Geometry check sheet. Reference: the model listing, model coordinates, mm. Face numbers are marked on the shaded views. A direction names the side the tool comes from. Coordinates: 2 decimals unless noted, no trailing zeros. Write each loop counter-clockwise with the first axis right and the second up, starting at its lowest first coordinate (ties: lowest second). Pieces come first, ordered by that corner, then holes. Notation, with made-up numbers: (-14.5, -18) -> (39.5, -18) arc R18 cw to (39.5, -2) -> close; hole circle Ø6 at (-39, 3.25). An arc over 180 degrees is marked (long way). Use a Markdown table: item, result.
```python
from build123d import *

# Parameters (mm, degrees)
SKETCH1_R                       = 1.975
PCB_DEPTH                       = 0.825
SKETCH7_R                       = 1.475
INNER_HOLES_DEPTH               = 1
INNER_HOLES_DEPTH_BACK          = 2.65
SKETCH8_W                       = 10
SKETCH8_H                       = 4.35
CONNECTOR_DEPTH                 = 2.6
SKETCH9_W                       = 4.3
SKETCH9_H                       = 2
TOP_COMPONENT_DEPTH             = 2.255
SKETCH10_W                      = 5.75
SKETCH10_H                      = 5
SIDE_COMPONENTS_DEPTH           = 1.1
SKETCH11_W                      = 10.5
SKETCH11_H                      = 17
CENTRAL_COMPONENTS_DEPTH        = 1.825
SKETCH12_W                      = 5.575
SKETCH12_H                      = 5
TOP_AND_BOTTOM_COMPONENTS_DEPTH = 1.105


with BuildPart() as part:
    # Sketch1 → PCB (new body, symmetric)
    with BuildSketch(Plane(origin=(0, 0, 0), x_dir=(1, 0, 0), z_dir=(0, 1, 0))):
        with BuildLine():
            Line((-7, 42.5), (7, 42.5))
            Line((7, 42.5), (7, 37))
            Line((7, 37), (14.725, 37))
            ThreePointArc((14.725, 37), (17.73020382, 35.75520382), (18.975, 32.75))
            Line((18.975, 32.75), (18.975, 31.75))
            Line((18.975, 31.75), (21.975, 31.75))
            Line((21.975, 31.75), (21.975, 5.25))
            Line((21.975, 5.25), (18.975, 5.25))
            Line((18.975, 5.25), (18.975, 4.25))
            ThreePointArc((18.975, 4.25), (17.73020382, 1.24479618), (14.725, 0))
            Line((14.725, 0), (-14.725, 0))
            ThreePointArc((-14.725, 0), (-17.73020382, 1.24479618), (-18.975, 4.25))
            Line((-18.975, 4.25), (-18.975, 5.25))
            Line((-18.975, 5.25), (-21.975, 5.25))
            Line((-21.975, 5.25), (-21.975, 31.75))
            Line((-21.975, 31.75), (-18.975, 31.75))
            Line((-18.975, 31.75), (-18.975, 32.75))
            ThreePointArc((-18.975, 32.75), (-17.73020382, 35.75520382), (-14.725, 37))
            Line((-14.725, 37), (-7, 37))
            Line((-7, 37), (-7, 42.5))
        make_face()
        with Locations((15.414429112, 33.439429112)):
            Circle(SKETCH1_R, mode=Mode.SUBTRACT)
        with Locations((15.414429112, 3.560570888)):
            Circle(SKETCH1_R, mode=Mode.SUBTRACT)
        with Locations((-15.414429112, 3.560570888)):
            Circle(SKETCH1_R, mode=Mode.SUBTRACT)
        with Locations((-15.414429112, 33.439429112)):
            Circle(SKETCH1_R, mode=Mode.SUBTRACT)
    extrude(amount=PCB_DEPTH, both=True)

    # Sketch7 → inner holes (cut, two sides)
    with BuildSketch(Plane(origin=(0, 0.825, 0), x_dir=(1, 0, 0), z_dir=(0, 1, 0))) as inner_holes_sk:
        with Locations((10.146483592, 28.171483592)):
            Circle(SKETCH7_R)
        with Locations((-10.146483592, 28.171483592)):
            Circle(SKETCH7_R)
        with Locations((-10.146483592, 8.828516408)):
            Circle(SKETCH7_R)
        with Locations((10.146483592, 8.828516408)):
            Circle(SKETCH7_R)
    extrude(amount=INNER_HOLES_DEPTH, mode=Mode.SUBTRACT)
    extrude(inner_holes_sk.sketch, amount=-INNER_HOLES_DEPTH_BACK, mode=Mode.SUBTRACT)

    # Sketch8 → Connector (add)
    with BuildSketch(Plane(origin=(0, 0.825, 0), x_dir=(1, 0, 0), z_dir=(0, 1, 0))):
        with Locations((0, 0.675)):
            Rectangle(SKETCH8_W, SKETCH8_H)
    extrude(amount=CONNECTOR_DEPTH)

    # Sketch9 → Top component (add)
    with BuildSketch(Plane(origin=(0, 0.825, 0), x_dir=(1, 0, 0), z_dir=(0, 1, 0))):
        with Locations((0, 36)):
            Rectangle(SKETCH9_W, SKETCH9_H)
    extrude(amount=TOP_COMPONENT_DEPTH)

    # Sketch10 → Side Components (add)
    with BuildSketch(Plane(origin=(0, 0.825, 0), x_dir=(1, 0, 0), z_dir=(0, 1, 0))):
        with Locations((15.53, 15.4)):
            Rectangle(SKETCH10_W, SKETCH10_H)
        with Locations((15.53, 9.2)):
            Rectangle(SKETCH10_W, SKETCH10_H)
        with Locations((15.53, 21.6)):
            Rectangle(SKETCH10_W, SKETCH10_H)
        with Locations((15.53, 27.8)):
            Rectangle(SKETCH10_W, SKETCH10_H)
        with Locations((-15.53, 9.2)):
            Rectangle(SKETCH10_W, SKETCH10_H)
        with Locations((-15.53, 15.4)):
            Rectangle(SKETCH10_W, SKETCH10_H)
        with Locations((-15.53, 21.6)):
            Rectangle(SKETCH10_W, SKETCH10_H)
        with Locations((-15.53, 27.8)):
            Rectangle(SKETCH10_W, SKETCH10_H)
    side_components = extrude(amount=SIDE_COMPONENTS_DEPTH)

    # Sketch11 → Central components (add)
    with BuildSketch(Plane(origin=(0, 0.825, 0), x_dir=(1, 0, 0), z_dir=(0, 1, 0))):
        with Locations((0, 18.5)):
            Rectangle(SKETCH11_W, SKETCH11_H)
    extrude(amount=CENTRAL_COMPONENTS_DEPTH)

    # Sketch12 → Top and bottom components (add)
    with BuildSketch(Plane(origin=(0, 0.825, 0), x_dir=(1, 0, 0), z_dir=(0, 1, 0))):
        with Locations((8.7625, 34.5)):
            Rectangle(SKETCH12_W, SKETCH12_H)
        with Locations((8.7625, 2.5)):
            Rectangle(SKETCH12_W, SKETCH12_H)
        with Locations((-8.7625, 2.5)):
            Rectangle(SKETCH12_W, SKETCH12_H)
        with Locations((-8.7625, 34.5)):
            Rectangle(SKETCH12_W, SKETCH12_H)
    top_and_bottom_components = extrude(amount=TOP_AND_BOTTOM_COMPONENTS_DEPTH)

    # Mirror2: Side Components, Top and bottom components across plane
    add(side_components.mirror(Plane.ZX))
    add(top_and_bottom_components.mirror(Plane.ZX))


solid = part.part
```
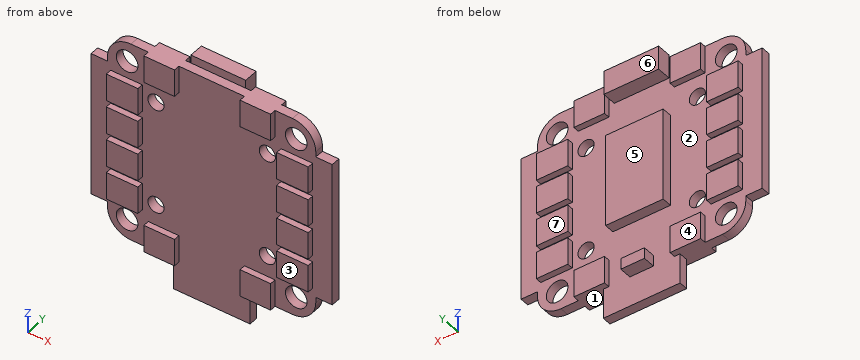
Item 1: Thickness scan on L1, parallel to Z at x = 17.5, y = 1.2; L2, parallel to Z at x = 1, y = 2.5; L3, parallel to X at y = 0.3, z = -5 (3 decimals). Record the ranges inside material, lowest first. Write a range as [from, to].
Answer block:
| item | result |
|---|---|
| L1 | z = [-30.3, -25.3], [-24.1, -19.1], [-17.9, -12.9], [-11.7, -6.7] |
| L2 | z = [-37, -35], [-27, -10], [-2.85, 1.5] |
| L3 | x = [-18.975, -16.767], [-14.062, 14.062], [16.767, 18.975] |
Item 2: Mould release check, pull along X, two halves, no side actions. Record for the marked faces 1 and 2: +X half, -X half, draft (parallel to the pull), parting line (faces both ways), or undercut.
Answer block:
| item | result |
|---|---|
| face 1 | draft |
| face 2 | undercut |
Item 3: Depth check by flat-ended pin: P1, Ø2.5, axis at x = 15, z = -14.5, coming from the +Y side (3 decimals); P2, Ø1, axis at y = 1.5, z = -36, coming from the +X side; P3, Ø0.8, axis at x = -20, y = 0, coming from the -Z side; P4, Ø3, axis at y = 2, z = -11, coming from the -X side (3 decimals). Enter the tip coordinate at first touch or a pass-through.
Answer block:
| item | result |
|---|---|
| P1 | stops at y = 1.925 |
| P2 | stops at x = 11.55 |
| P3 | stops at z = -31.75 |
| P4 | stops at x = -21.975 |
Item 4: Section check C-C on x = 9.5. Record the boundary of the cut face in (y, z) (3 decimals), then the cut area to 3 significant figures.
Answer block:
| item | result |
|---|---|
| outline | (-1.93, -37) -> (1.93, -37) -> (1.93, -32) -> (0.825, -32) -> (0.825, -29.497) -> (-0.825, -29.497) -> (-0.825, -32) -> (-1.93, -32) -> close; (-1.93, -5) -> (-0.825, -5) -> (-0.825, -7.503) -> (0.825, -7.503) -> (0.825, -5) -> (1.93, -5) -> (1.93, 0) -> (-1.93, 0) -> close; (-0.825, -26.846) -> (0.825, -26.846) -> (0.825, -10.154) -> (-0.825, -10.154) -> close |
| area | 74.4 mm^2 |
Item 5: Section check A-A on x = -3. Record the boundary of the cut face in (y, z) (3 decimals), then the cut area to 3 significant figures.
Answer block:
| item | result |
|---|---|
| outline | (-0.825, -42.5) -> (0.825, -42.5) -> (0.825, -27) -> (2.65, -27) -> (2.65, -10) -> (0.825, -10) -> (0.825, -2.85) -> (3.425, -2.85) -> (3.425, 1.5) -> (0.825, 1.5) -> (0.825, 0) -> (-0.825, 0) -> close |
| area | 112 mm^2 |
Item 6: Section check B-B on z = -34.5. Count the separate pieces of the cut face and the enclosed holes in it, then the cut area to 3 significant figures.
Answer block:
| item | result |
|---|---|
| separate pieces | 3 |
| enclosed holes | 0 |
| area | 75.0 mm^2 |
Item 7: Tool access check on the marked faces 3, 4, 5, 6 and 7. Record the directions out of +Z, -Z, +X, -X, +Y, -Y that give a thin tool (end or side, any length) a straight path to the whole face; none if there is none.
Answer block:
| item | result |
|---|---|
| face 3 | +Z, -Z, +X, -X, -Y |
| face 4 | +Z, -Z, -X, +Y |
| face 5 | +X, -X, +Y |
| face 6 | +Z, -Z, +X, -X, +Y |
| face 7 | +Z, -Z, +X, +Y |
